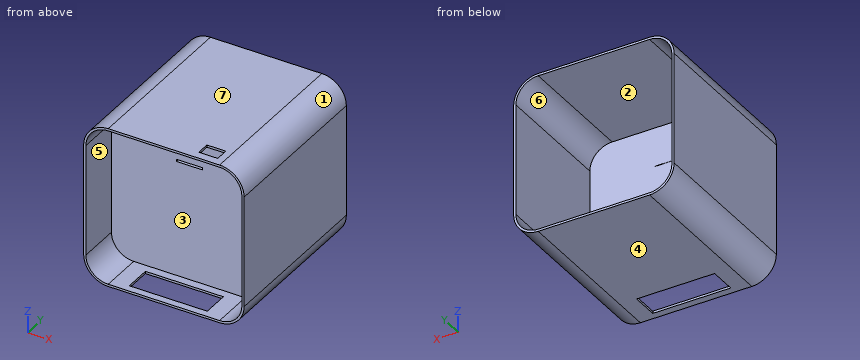
```python
from build123d import *

# Parameters (mm, degrees)
ESQUISSE1_W             = 140
ESQUISSE1_H             = 140
BOSS_EXTRU_1_DEPTH      = 150
CONG_1_R                = 20
COQUE1_T                = 2
BOSS_EXTRU_2_START      = 40
BOSS_EXTRU_2_DEPTH      = 40
ENL_V_START             = -38
ENL_V_MAT_EXTRU_1_DEPTH = 38
ESQUISSE4_W             = 23
ESQUISSE4_H             = 2
ENL_V_MAT_EXTRU_2_DEPTH = 33
ESQUISSE5_W             = 70
ESQUISSE5_H             = 24
ENL_V_MAT_EXTRU_3_DEPTH = 33
ESQUISSE6_W             = 17
ESQUISSE6_H             = 12
ENL_V_MAT_EXTRU_4_DEPTH = 33
BOSS_EXTRU_3_DEPTH      = 23
BOSS_EXTRU_4_DEPTH      = 23
ESQUISSE12_R            = 1.475
BOSS_EXTRU_5_DEPTH      = 3


with BuildPart() as part:
    # Esquisse1 → Boss.-Extru.1 (new body)
    with BuildSketch(Plane(origin=(0, 0, 0), x_dir=(1, 0, 0), z_dir=(0, 1, 0))):
        Rectangle(ESQUISSE1_W, ESQUISSE1_H)
    extrude(amount=BOSS_EXTRU_1_DEPTH)

    # Congé1
    cong_1_edges = [part.edges().sort_by_distance(p)[0] for p in [
        (70, 75, 70),
        (-70, 75, 70),
        (-70, 75, -70),
        (70, 75, -70),
    ]]
    fillet(cong_1_edges, radius=CONG_1_R)

    # Coque1
    coque1_openings = [part.faces().sort_by_distance(p)[0] for p in [
        (0, 150, 0),
    ]]
    offset(amount=COQUE1_T, openings=coque1_openings, kind=Kind.INTERSECTION)

    # Esquisse2 → Boss.-Extru.2 (add)
    with BuildSketch(Plane(origin=(0, 0, 0), x_dir=(1, 0, 0), z_dir=(0, 1, 0)).offset(BOSS_EXTRU_2_START)):
        with BuildLine():
            Line((70, -50), (70, 50))
            ThreePointArc((70, 50), (64.142135624, 64.142135624), (50, 70))
            Line((50, 70), (-50, 70))
            ThreePointArc((-50, 70), (-64.142135624, 64.142135624), (-70, 50))
            Line((-70, 50), (-70, -50))
            ThreePointArc((-70, -50), (-64.142135624, -64.142135624), (-50, -70))
            Line((-50, -70), (50, -70))
            ThreePointArc((50, -70), (64.142135624, -64.142135624), (70, -50))
        make_face()
    extrude(amount=-BOSS_EXTRU_2_DEPTH)

    # Esquisse3 → Enlèv. mat.-Extru.1 (cut)
    with BuildSketch(Plane.XZ.offset(2).offset(ENL_V_START)):
        with BuildLine():
            Line((70, -50), (70, 50))
            ThreePointArc((70, 50), (64.142135624, 64.142135624), (50, 70))
            Line((50, 70), (-50, 70))
            ThreePointArc((-50, 70), (-64.142135624, 64.142135624), (-70, 50))
            Line((-70, 50), (-70, -50))
            ThreePointArc((-70, -50), (-64.142135624, -64.142135624), (-50, -70))
            Line((-50, -70), (50, -70))
            ThreePointArc((50, -70), (64.142135624, -64.142135624), (70, -50))
        make_face()
    extrude(amount=ENL_V_MAT_EXTRU_1_DEPTH, mode=Mode.SUBTRACT)

    # Esquisse4 → Enlèv. mat.-Extru.2 (cut)
    with BuildSketch(Plane.XZ.offset(-36)):
        with Locations((0, 34.941356373)):
            Rectangle(ESQUISSE4_W, ESQUISSE4_H)
    extrude(amount=-ENL_V_MAT_EXTRU_2_DEPTH, mode=Mode.SUBTRACT)

    # Esquisse5 → Enlèv. mat.-Extru.3 (cut)
    with BuildSketch(Plane(origin=(0, 0, -72), x_dir=(-1, 0, 0), z_dir=(0, 0, -1))):
        with Locations((0, 16.5)):
            Rectangle(ESQUISSE5_W, ESQUISSE5_H)
    extrude(amount=-ENL_V_MAT_EXTRU_3_DEPTH, mode=Mode.SUBTRACT)

    # Esquisse6 → Enlèv. mat.-Extru.4 (cut)
    with BuildSketch(Plane.XY.offset(72)):
        with Locations((35.41933702, 11.338578381)):
            Rectangle(ESQUISSE6_W, ESQUISSE6_H)
    extrude(amount=-ENL_V_MAT_EXTRU_4_DEPTH, mode=Mode.SUBTRACT)

    # Esquisse7 → Boss.-Extru.3 (add)
    with BuildSketch(Plane.ZY.offset(-11.5)):
        Polygon((33.941356373, 40), (34.841356373, 40), (34.841356373, 39.856828703), (33.941356373, 39.75), align=None)
    extrude(amount=BOSS_EXTRU_3_DEPTH)

    # Esquisse10 → Boss.-Extru.4 (add)
    with BuildSketch(Plane(origin=(-11.5, 0, 0), x_dir=(0, 0, -1), z_dir=(1, 0, 0))):
        Polygon((-35.941356373, 40), (-35.041356373, 40), (-35.041356373, 39.885374009), (-35.941356373, 39.75), align=None)
    extrude(amount=BOSS_EXTRU_4_DEPTH)

    # Esquisse12 → Boss.-Extru.5 (add)
    with BuildSketch(Plane(origin=(0, 0, 70), x_dir=(-1, 0, 0), z_dir=(0, 0, -1))):
        with Locations(Location((28.043934099, 18.476473505, 0), (0, 0, 180))):
            Circle(ESQUISSE12_R)
    extrude(amount=BOSS_EXTRU_5_DEPTH)


solid = part.part
```
CAD build for the part. Positions are in the model's coordinates, mm. Face numbers are marked on the shaded views. A direction names the side the tool comes from. Round coordinates to 2 decimals unless told otherwise and drop trailing zeros. Loops run counter-clockwise (first coordinate to the right, second up) from the corner with the lowest first, then second, coordinate; pieces in that order, holes last. Notation, with made-up numbers: (58, 45) - (67, 45) arc R10 cw to (67, 59) - close; hole circle Ø1 at (-8.5, 45). An arc over 180 degrees is marked (long way). Return JSON: item names as keys, results as strings. Group by question number.
Q1. Band-saw the part on B-B on x = -23. Give the cut face in (y, z).
Q2. Flat gauge pins, fed straight in: pin 1 Ø11.5 at (x, y) = (11.5, 14) entering from -Z; pin 2 Ø1.6 at (y, z) = (8.5, 71) entering from -X; pin 3 Ø3 at (x, y) = (-56, 85.5) entering from +Z. Where does each tip first touch, or does it go through?
Q3. Two-plate mould, pull along Z, no slides. Class the marked faces 1, 2, 3 and 4: +Z half, -Z half, draft (parallel to the pull), parting line (faces both ways), or undercut.
Q4. Band-saw the part on C-C on x = -44. Give the cut face in (y, z).
Q5. Band-saw the part on A-A on y = 56.5. Give the cut face in (x, z), plus the area to 3 significant figures.
Q6. Drill centre lines: line 1 along X through (y, z) = (86, -50.5); line 2 along Z through (x, y) = (-32, 32.5); line 3 along Y through (x, z) = (39, -65.5). Where is each one in solid material? Low to high. Write a range as [from, to].
Q7. Band-saw the part on D-D on z = -42. Give the cut face in (x, y), plus the area to 3 significant figures.
Q8. Tool access for the marked faces 5, 6 and 7: list every direction of +Z, -Z, +X, -X, +Y, -Y with a clear straight run to the whole face (end or side of a thin tool).
Solutions:
{
 "1": {"outline": "(-2, -72) - (4.5, -72) - (4.5, -70) - (-2, -70) - close; (-2, 70) - (36, 70) - (36, -70) - (28.5, -70) - (28.5, -72) - (150, -72) - (150, -70) - (40, -70) - (40, 70) - (150, 70) - (150, 72) - (-2, 72) - close"},
 "2": {"pin 1": "stops at z = 70", "pin 2": "stops at x = -58.72", "pin 3": "stops at z = 71.53"},
 "3": {"face 1": "+Z half", "face 2": "undercut", "face 3": "undercut", "face 4": "-Z half"},
 "4": {"outline": "(-2, -72) - (150, -72) - (150, -70) - (40, -70) - (40, 70) - (150, 70) - (150, 72) - (-2, 72) - (-2, 70) - (36, 70) - (36, -70) - (-2, -70) - close"},
 "5": {"outline": "(-72, -50) arc R22 ccw to (-50, -72) - (50, -72) arc R22 ccw to (72, -50) - (72, 50) arc R22 ccw to (50, 72) - (-50, 72) arc R22 ccw to (-72, 50) - close; hole (-70, -50) arc R20 ccw to (-50, -70) - (50, -70) arc R20 ccw to (70, -50) - (70, 50) arc R20 ccw to (50, 70) - (-50, 70) arc R20 ccw to (-70, 50) - close", "area": "1,060 mm^2"},
 "6": {"line 1": "x = [-71.99, -69.99], [69.99, 71.99]", "line 2": "z = [-72, -70], [70, 72]", "line 3": "y = [36, 40]"},
 "7": {"outline": "(-72, -2) - (-70, -2) - (-70, 36) - (70, 36) - (70, -2) - (72, -2) - (72, 150) - (70, 150) - (70, 40) - (-70, 40) - (-70, 150) - (-72, 150) - close", "area": "1,170 mm^2"},
 "8": {"face 5": "-Y", "face 6": "+Y", "face 7": "+Z, +X, -X, +Y, -Y"}
}
